Check sheet for the modelled part. Datum: model origin and axes. Units: mm. Give positions to 0.01 mm unless a question says otherwise; leave off trailing zeros. Order: outer loops, then holes, each group sorted by start corner. A loop starts at its lowest first (then second) coordinate and runs counter-clockwise, first axis right, second up.
from build123d import *

# Parameters (mm, degrees)
SKETCH1_W           = 863.6
SKETCH1_H           = 558.8
BOSS_EXTRUDE1_DEPTH = 7.62
CHAMFER1_SIZE       = 203.2
CHAMFER2_SIZE       = 203.2
CHAMFER3_SIZE       = 203.2
CHAMFER4_SIZE       = 203.2


with BuildPart() as part:
    # Sketch1 → Boss-Extrude1 (new body)
    with BuildSketch(Plane.XY):
        with Locations((7.119883608, -41.512124151)):
            Rectangle(SKETCH1_W, SKETCH1_H)
    extrude(amount=BOSS_EXTRUDE1_DEPTH)

    # Chamfer1
    chamfer1_edges = [part.edges().sort_by_distance(p)[0] for p in [
        (-424.680116392, 237.887875849, 3.81),
    ]]
    chamfer(chamfer1_edges, length=CHAMFER1_SIZE)

    # Chamfer2
    chamfer2_edges = [part.edges().sort_by_distance(p)[0] for p in [
        (-424.680116392, -320.912124151, 3.81),
    ]]
    chamfer(chamfer2_edges, length=CHAMFER2_SIZE)

    # Chamfer3
    chamfer3_edges = [part.edges().sort_by_distance(p)[0] for p in [
        (438.919883608, -320.912124151, 3.81),
    ]]
    chamfer(chamfer3_edges, length=CHAMFER3_SIZE)

    # Chamfer4
    chamfer4_edges = [part.edges().sort_by_distance(p)[0] for p in [
        (438.919883608, 237.887875849, 3.81),
    ]]
    chamfer(chamfer4_edges, length=CHAMFER4_SIZE)


solid = part.part
1) Section check B-B, the plane x = -345. Record the cut outline in (y, z), then the cut area to 3 significant figures.
Recorded:
outline: (-197.39, 0) - (114.37, 0) - (114.37, 7.62) - (-197.39, 7.62) - close
area: 2,380 mm2
2) Section check C-C, the plane y = -274. Record the cut outline in (x, z).
Recorded:
outline: (-268.39, 0) - (282.63, 0) - (282.63, 7.62) - (-268.39, 7.62) - close
3) Section check A-A, the plane z = 2.5. Record the cut outline in (x, y).
Recorded:
outline: (-424.68, -117.71) - (-221.48, -320.91) - (235.72, -320.91) - (438.92, -117.71) - (438.92, 34.69) - (235.72, 237.89) - (-221.48, 237.89) - (-424.68, 34.69) - close
4) Depth check by flat-ended pin: pin 1 Ø4 at (y, z) = (135, 2.5) entering from +X; pin 2 Ø3 at (x, z) = (286, 2.5) entering from +Y. Enter the tip coordinate at first touch or a pass-through.
Recorded:
pin 1: stops at x = 340.61
pin 2: stops at y = 189.11
5) Material ranges on L1, parallel to Y at x = -364.5, z = 0.5; L2, parallel to X at y = -238.5, z = 1; L3, parallel to Y at x = -240, z = 6.25, recorded low to high.
Recorded:
L1: y = -177.89 to 94.87
L2: x = -303.89 to 318.13
L3: y = -302.39 to 219.37
